Geometry check sheet. Reference: the model listing, model coordinates, mm. Face numbers are marked on the shaded views. Give positions to 0.01 mm unless a question says otherwise; leave off trailing zeros. Loops run counter-clockwise (first coordinate to the right, second up) from the corner with the lowest first, then second, coordinate; pieces in that order, holes last. Notation, with made-up numbers: (0, 69) -> (6, 69) arc R35 ccw to (6, 107) -> close; hole circle Ø1 at (38.5, 65). An arc over 180 degrees is marked (long way). Write each question's results on one line, items separated by ' | '. Start each with the question number.
1) Sectioned sample at D-D on y = 26.5. Record the cut outline in (x, z).
2) Sectioned sample at C-C on x = 15. Record the cut outline in (y, z).
3) Scan lines: line 1 (X direction, y = 6, z = 1.8); line 2 (Z direction, x = 11.5, y = 10.5); line 3 (Y direction, x = 4, z = 1.75). Record each from-to range of solid material in increasing order. Write a range as from..to.
4) Depth check by flat-ended pin: pin 1 (1.5 mm diameter, centred on x = 4.5, z = 1.5, fed in from +Y); pin 2 (2 mm diameter, centred on x = 6, y = 37, fed in from -Z); pin 3 (1.5 mm diameter, centred on y = 44, z = 2, fed in from +X) (3 decimals); pin 4 (1.5 mm diameter, centred on y = 41.5, z = 1.5, fed in from -X) (3 decimals). Enter the tip coordinate at first touch or a pass-through.
5) Sectioned sample at A-A on y = 20. Record the cut outline in (x, z).
6) Draft check along X on the marked faces 1, 2, 3 and 4. Enter one of: pulls with the +X half, pulls with the -X half, needs draft (parallel to the pull), parting line crosses it, or undercut.
```python
from build123d import *

# Parameters (mm, degrees)
BOSS_EXTRUDE1_DEPTH = 3
CUT_EXTRUDE1_DEPTH  = 2.2
SKETCH3_R           = 2.875
CUT_EXTRUDE2_DEPTH  = 22.6
CUT_EXTRUDE3_DEPTH  = 2.2
FILLET1_R           = 2
FILLET2_R           = 4
FILLET3_R           = 4
SKETCH5_W           = 7.5
SKETCH5_H           = 7.5
CUT_EXTRUDE4_DEPTH  = 0.8
FILLET4_R           = 1


with BuildPart() as part:
    # Sketch1 → Boss-Extrude1 (new body)
    with BuildSketch(Plane.XY):
        Polygon((0, 36), (9.325, 36), (9.325, 46), (16.675, 46), (16.675, 36), (26, 36), (26, 0), (0, 0), align=None)
    extrude(amount=BOSS_EXTRUDE1_DEPTH)

    # Sketch2 → Cut-Extrude1 (cut)
    with BuildSketch(Plane.XY.offset(3)):
        with BuildLine():
            Line((1.1, -0.4), (1.1, 0.795839104))
            ThreePointArc((1.1, 0.795839104), (2.1, 2.3), (1.1, 3.804160896))
            Line((1.1, 3.804160896), (1.1, 23.4))
            Line((1.1, 23.4), (24.9, 23.4))
            Line((24.9, 23.4), (24.9, 3.804160896))
            ThreePointArc((24.9, 3.804160896), (23.9, 2.3), (24.9, 0.795839104))
            Line((24.9, 0.795839104), (24.9, -0.4))
            Line((24.9, -0.4), (1.1, -0.4))
        make_face()
    extrude(amount=-CUT_EXTRUDE1_DEPTH, mode=Mode.SUBTRACT)

    # Sketch3 → Cut-Extrude2 (cut)
    with BuildSketch(Plane(origin=(0, 46, 0), x_dir=(1, 0, 0), z_dir=(0, 1, 0))):
        with Locations((13, -3.675)):
            Circle(SKETCH3_R)
    extrude(amount=-CUT_EXTRUDE2_DEPTH, mode=Mode.SUBTRACT)

    # Sketch4 → Cut-Extrude3 (cut)
    with BuildSketch(Plane.XY.offset(3)):
        Polygon((5.652681139, 23.4), (10.205362278, 34.7), (15.794637722, 34.7), (20.347318861, 23.4), align=None)
    extrude(amount=-CUT_EXTRUDE3_DEPTH, mode=Mode.SUBTRACT)

    # Fillet1
    fillet1_edges = [part.edges().sort_by_distance(p)[0] for p in [
        (10.205362278, 34.7, 1.9),
        (20.347318861, 23.4, 1.9),
        (15.794637722, 34.7, 1.9),
        (5.652681139, 23.4, 1.9),
    ]]
    fillet(fillet1_edges, radius=FILLET1_R)

    # Fillet2
    fillet2_edges = [part.edges().sort_by_distance(p)[0] for p in [
        (0, 36, 1.5),
        (26, 36, 1.5),
    ]]
    fillet(fillet2_edges, radius=FILLET2_R)

    # Fillet3
    fillet3_edges = [part.edges().sort_by_distance(p)[0] for p in [
        (9.325, 36, 1.5),
        (16.675, 36, 1.5),
    ]]
    fillet(fillet3_edges, radius=FILLET3_R)

    # Sketch5 → Cut-Extrude4 (cut)
    with BuildSketch(Plane.XY.offset(0.8)):
        with Locations((13, 19.65)):
            Rectangle(SKETCH5_W, SKETCH5_H)
    extrude(amount=-CUT_EXTRUDE4_DEPTH, mode=Mode.SUBTRACT)

    # Fillet4
    fillet4_edges = [part.edges().sort_by_distance(p)[0] for p in [
        (16.75, 15.9, 0.4),
        (16.75, 23.4, 0.4),
        (9.25, 23.4, 0.4),
        (9.25, 15.9, 0.4),
    ]]
    fillet(fillet4_edges, radius=FILLET4_R)


solid = part.part
```
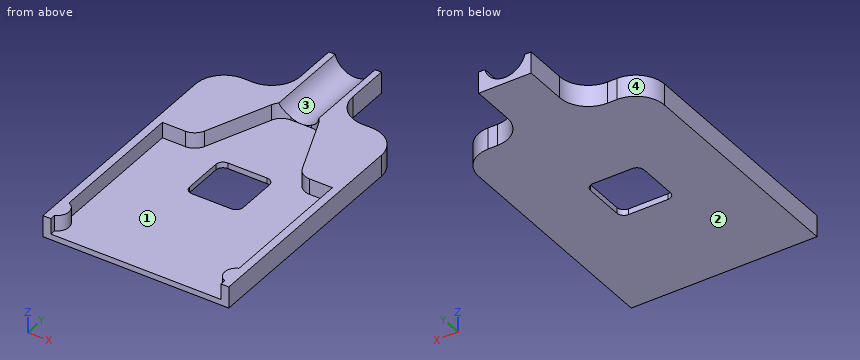
Result:
1) outline: (0, 0) -> (26, 0) -> (26, 3) -> (19.1, 3) -> (19.1, 0.8) -> (6.9, 0.8) -> (6.9, 3) -> (0, 3) -> close
2) outline: (0, 0) -> (15.9, 0) -> (15.9, 0.8) -> (0, 0.8) -> close; (23.4, 0) -> (46, 0) -> (46, 1.61) -> (34.62, 1.61) -> (34.62, 0.8) -> (23.4, 0.8) -> close
3) line 1: 0..1.1, 24.9..26 | line 2: 0..0.8 | line 3: 23.4..36
4) pin 1: y = 36 | pin 2: z = 0 | pin 3: x = 16.675 | pin 4: x = 9.325
5) outline: (0, 0) -> (9.25, 0) -> (9.25, 0.8) -> (1.1, 0.8) -> (1.1, 3) -> (0, 3) -> close; (16.75, 0) -> (26, 0) -> (26, 3) -> (24.9, 3) -> (24.9, 0.8) -> (16.75, 0.8) -> close
6) face 1: undercut | face 2: needs draft | face 3: undercut | face 4: pulls with the -X half
